Here's the drawing with two shaded views (mm, measured from the low corner). I have some questions. A direction names the side the tool comes from. Coordinates: 2 decimals unless noted, no trailing zeros. Order: outer loops, then holes, each group sorted by start corner. A loop starts at its lowest first (then second) coordinate and runs counter-clockwise, first axis right, second up. Notation, with made-up numbers: (86, 52) -> (95, 52) arc R18 ccw to (95, 63) -> close; hole circle Ø3 at (84, -32.75). An arc over 180 degrees is marked (long way). Answer as a JSON object with one key per item and string values. Group by question number.
(1) If we mould it in two halves opening along X, with no side actions, what happens to the marked faces 1, 2 and 3? For each: pulls with the +X half, pulls with the -X half, needs draft (parallel to the pull), parting line crosses it, or undercut.
(2) For pin 1 (1.5 mm diameter, centred on x = 12.5, z = 23.5, fed in from +Y) (1 decimal); pin 2 (1 mm diameter, centred on x = 47.5, z = 33.5, fed in from +Y) (1 decimal); pin 3 (3 mm diameter, centred on y = 40.5, z = 20, fed in from +X); pin 4 (3 mm diameter, centred on x = 74, y = 11.5, fed in from -Z), each with a flat end and sliding along its axis, tell me the tip position at first contact or that it passes through.
(3) I want a section at A-A, the plane z = 27.5. List the corners of the cut face in (x, y) for me (1 decimal), plus the area to 3 significant figures.
(4) I need wall thicknesses on line 1 (X direction, y = 42, z = 40) (1 decimal); line 2 (Z direction, x = 70, y = 59.5); line 3 (Z direction, x = 90, y = 64.5). Which ranges of each line are inside material? Lowest first, please.
(5) Which directions (+Z, -Z, +X, -X, +Y, -Y) give clear straight access to the entire face, cutting with the end or side of a thin tool? Please do the marked faces 4, 5 and 6.
(6) I want a section at B-B, the plane z = 14. List the corners of the cut face in (x, y) for me (1 decimal).
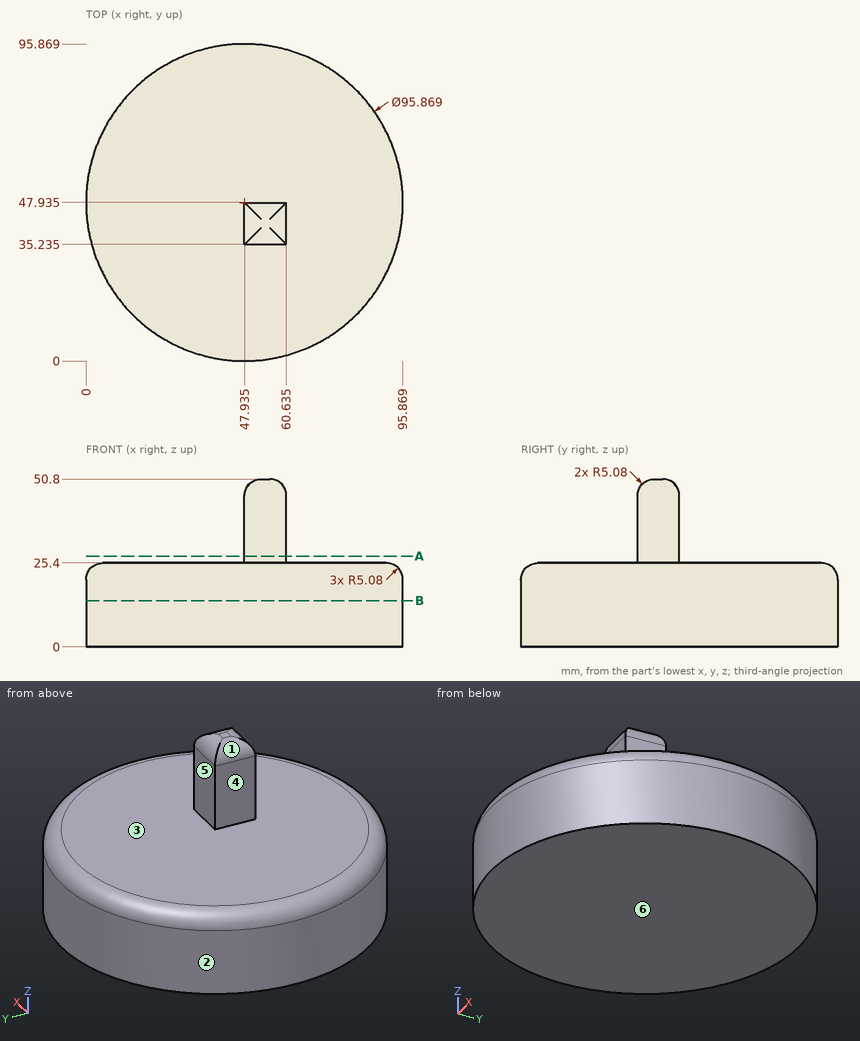
Computed values:
{
 "1": {"face 1": "pulls with the -X half", "face 2": "parting line crosses it", "face 3": "needs draft"},
 "2": {"pin 1": "stops at y = 79.7", "pin 2": "stops at y = 47.9", "pin 3": "stops at x = 95.5", "pin 4": "stops at z = 0"},
 "3": {"outline": "(47.9, 35.2) -> (60.6, 35.2) -> (60.6, 47.9) -> (47.9, 47.9) -> close", "area": "161 mm2"},
 "4": {"line 1": "x = 47.9 to 60.6", "line 2": "z = 0 to 25.4", "line 3": "z = 0 to 24.82"},
 "5": {"face 4": "+Z, -X, +Y, -Y", "face 5": "+Z, +X, -X, +Y", "face 6": "-Z, +X, -X, +Y, -Y"},
 "6": {"outline": "circle Ø95.9 at (47.9, 47.9)"}
}
